```python
from build123d import *

# Parameters (mm, degrees)
SKIZZE1_W                                 = 25
SKIZZE1_H                                 = 24
PCB_DEPTH                                 = 0.9
SKIZZE2_R                                 = 1.05
MOUNTING_HOLES_DEPTH                      = 20.165333287
SKIZZE3_W                                 = 20.8
SKIZZE3_H                                 = 5.5
CONNECTOR_CLOSED_DEPTH                    = 2.4
SKIZZE4_W                                 = 17.7
SKIZZE4_H                                 = 11.6
COMPONENTS_WORST_CASE_BOUNDARY_BOX_DEPTH  = 1.3
SKIZZE6_W                                 = 16
SKIZZE6_H                                 = 0.4
SKIZZE7_W                                 = 3
SKIZZE7_H                                 = 2
COMPONENTS_WORST_CASE_BOUNDARY_BOX2_DEPTH = 0.6
SKIZZE8_W                                 = 1.3
SKIZZE8_H                                 = 0.9
STATUS_LED_DEPTH                          = 0.01


with BuildPart() as part:
    # Skizze1 → PCB (new body)
    with BuildSketch(Plane(origin=(0, 0, 0), x_dir=(1, 0, 0), z_dir=(0, 1, 0))):
        with Locations((0, 2.5)):
            Rectangle(SKIZZE1_W, SKIZZE1_H)
    extrude(amount=-PCB_DEPTH)

    # Skizze2 → Mounting_Holes (cut, through all)
    with BuildSketch(Plane(origin=(0, 0, 0), x_dir=(1, 0, 0), z_dir=(0, 1, 0))):
        with Locations(Location((10.5, 12.5, 0), (0, 0, 270))):
            Circle(SKIZZE2_R)
        with Locations(Location((10.5, 0, 0), (0, 0, 270))):
            Circle(SKIZZE2_R)
        with Locations(Location((-10.5, 0, 0), (0, 0, 90))):
            Circle(SKIZZE2_R)
        with Locations(Location((-10.5, 12.5, 0), (0, 0, 90))):
            Circle(SKIZZE2_R)
    extrude(amount=-MOUNTING_HOLES_DEPTH, mode=Mode.SUBTRACT)

    # Skizze3 → Connector_closed (add)
    with BuildSketch(Plane.XZ.offset(0.9)):
        with Locations((0, 6.75)):
            Rectangle(SKIZZE3_W, SKIZZE3_H)
    extrude(amount=CONNECTOR_CLOSED_DEPTH)

    # Skizze4 → Components_worst-case_Boundary-Box (add)
    with BuildSketch(Plane.XZ.offset(0.9)):
        with Locations((-0.15, -6.7)):
            Rectangle(SKIZZE4_W, SKIZZE4_H)
    extrude(amount=COMPONENTS_WORST_CASE_BOUNDARY_BOX_DEPTH)

    # Cable_156mm_free_Length: sweep along a path in Skizze5
    with BuildLine() as cable_156mm_free_length_path:  # in the path sketch's own coordinates; laid on its plane below (add() does not lay a ready-made edge on the line's plane)
        Line((-133.7358537, -42.734939928), (-127.749991329, -42.323294834))
        add(Edge.make_bspline(
            [(-127.749991329, -42.323294834), (-47.264941103, -36.788373718), (-57.962969562, -2.1), (-9.5, -2.1)],
            knots=[0, 0, 0, 0, 1, 1, 1, 1], degree=3))
    # Skizze6 → Cable_156mm_free_Length (sweep)
    with BuildSketch(Plane.XY.offset(9.5)):
        with Locations((0, -2.3)):
            Rectangle(SKIZZE6_W, SKIZZE6_H)
    sweep(path=Plane(origin=(0, 0, 0), x_dir=(0, 0, -1), z_dir=(1, 0, 0)) * cable_156mm_free_length_path.line)

    # Skizze7 → Components_worst-case_Boundary-Box2 (add)
    with BuildSketch(Plane(origin=(0, 0, 0), x_dir=(1, 0, 0), z_dir=(0, 1, 0))):
        with Locations((7, 9.9)):
            Rectangle(SKIZZE7_W, SKIZZE7_H)
    extrude(amount=COMPONENTS_WORST_CASE_BOUNDARY_BOX2_DEPTH)

    # Skizze8 → Status_LED (cut)
    with BuildSketch(Plane(origin=(0, 0.6, 0), x_dir=(1, 0, 0), z_dir=(0, 1, 0))):
        with Locations((7.45, 9.45)):
            Rectangle(SKIZZE8_W, SKIZZE8_H)
    extrude(amount=-STATUS_LED_DEPTH, mode=Mode.SUBTRACT)


solid = part.part
```
For this review, take the finished solid that the model builds, in its own axes (mm). A direction names the side the tool comes from. Round coordinates to 2 decimals unless told otherwise and drop trailing zeros. One line per item, written item: value. Start each with the question number.
(1) Machinability: for faces 4 (the flat face through (10.4, -2, 7)), 5 (the flat face through (0, -2.2, -7)), 6 (the flat face through (0, -2, 4)), which of the approach directions +Z, -Z, +X, -X, +Y, -Y give a long, thin tool a straight path to every point of the face, cutting with its end or side? Answer none if there is none.
(2) Wall thickness on line 1 (X direction, y = -0.4, z = -12.5); line 2 (Z direction, x = -10.5, y = -0.5); line 3 (Y direction, x = 3.75, z = 0): over which ranges is each line inside the solid? List them lowest first.
(3) The part is to be moulded in two halves that separate along Z. For faces 1 (the flat face through (-10.4, -2, 7)), 2 (the flat face through (0.112, -42.526, 130.701)), 3 (the flat face through (-0.2, -1.6, 9.5)), say which applies: released by +Z, released by -Z, zero draft, split by the parting line, or undercut.
(4) Insertion check: pin 1 (3 mm diameter, centred on x = 3.5, z = 89.5, fed in from +Y); pin 2 (12 mm diameter, centred on x = -1, z = -6, fed in from +Y); pin 3 (1 mm diameter, centred on x = 4, y = -1.5, fed in from +Z). Each pin has a flat end and moves straight along its axis. Give the tip position at first contact, or say it passes through.
Result:
1. face 4: +Z, -Z, +X, -Y
1. face 5: -Z, +X, -X, -Y
1. face 6: +X, -X, -Y
2. line 1: -12.5 to -11.55, -9.45 to 9.45, 11.55 to 12.5
2. line 2: -14.5 to -13.55, -11.45 to -1.05, 1.05 to 9.5
2. line 3: -0.9 to 0
3. face 1: zero draft
3. face 2: released by +Z
3. face 3: undercut
4. pin 1: y = -35.66
4. pin 2: y = 0
4. pin 3: z = 9.5
